The listing builds one solid part. Answer for the finished solid, in the listing's coordinates (mm). A direction names the side the tool comes from. Give positions to 0.01 mm unless a question says otherwise; leave off trailing zeros. Loops run counter-clockwise (first coordinate to the right, second up) from the corner with the lowest first, then second, coordinate; pieces in that order, holes last.
Item 1: Each of these flat-tipped pins is pushed along its axis until it touches: pin 1 Ø6 at (x, z) = (-109, 26.5) entering from -Y; pin 2 Ø10 at (x, y) = (-134.5, 146) entering from +Z; pin 3 Ø6.5 at (y, z) = (-149.5, 4.5) entering from +X. Where does it stop, or does it pass through?
Item 2: Section C-C, the plane x = 77 is taken. Give the vertices of the cut face in (y, z).
Item 3: A tool of negligible diameter and unlimited length cuts with its end or side. For faces 4 (the face through (12.7, 149, 6)), 5 (the face through (-2, -117, -25.4)), 6 (the face through (-2, 118, -25.4)), 7 (the face through (-91.315, -114.144, -12.522)), from which of +Z, -Z, +X, -X, +Y, -Y can it reach the whole face along a straight path? Write none if from no direction.
Item 4: Consider line 1 along Z through (x, y) = (-161, 0); line 2 along Y through (x, z) = (-107.5, 90.5); line 3 along Y through (x, z) = (-145, 133). Determine where each line is inside the solid, lowest interval first.
Item 5: Section A-A, the plane z = 133.35 is taken. Give the vertices of the cut face in (x, y), and give its area (3 significant figures).
Item 6: Section D-D, the plane y = 0 is taken. Give the vertices of the cut face in (x, z).
Item 7: The mould has two halves that part along X. Classify faces 1 (the face through (-58.1, -149.4, 83.5)), 2 (the face through (156.335, -114.144, -12.522)), 3 (the face through (-82, -158.75, 58)): pulls with the +X half, pulls with the -X half, needs draft (parallel to the pull), parting line crosses it, or undercut.
Item 8: Section B-B, the plane y = 114.3 is taken. Give the vertices of the cut face in (x, z).
from build123d import *

# Parameters (mm, degrees)
F0_W           = 342.9
F0_H           = 330.2
F1_DEPTH       = 25.4
F2_W           = 342.9
F2_H           = 139.7
F3_DEPTH       = 6.35
F4_W           = 25.4
F4_H           = 304.8
F5_DEPTH       = 215.9
F7_D           = 127
F7_CBORE_D     = 139.7
F7_CBORE_DEPTH = 12.7
F9_DEPTH       = 1.524
F11_D          = 10.71626
F12_W          = 152.4
F12_H          = 19.05
F13_DEPTH      = 152.4
F14_SIZE       = 139.7


with BuildPart() as f1:
    # F0 (on Top) → F1 (new body)
    with BuildSketch(Plane.XY):
        Rectangle(F0_W, F0_H)
        with BuildLine():
            Line((-98.425, -121.412), (-117.475, -121.412))
            ThreePointArc((-117.475, -121.412), (-124.587, -114.3), (-117.475, -107.188))
            Line((-117.475, -107.188), (-98.425, -107.188))
            ThreePointArc((-98.425, -107.188), (-91.313, -114.3), (-98.425, -121.412))
        make_face(mode=Mode.SUBTRACT)
        with BuildLine():
            Line((149.225, -121.412), (130.175, -121.412))
            ThreePointArc((130.175, -121.412), (123.063, -114.3), (130.175, -107.188))
            Line((130.175, -107.188), (149.225, -107.188))
            ThreePointArc((149.225, -107.188), (156.337, -114.3), (149.225, -121.412))
        make_face(mode=Mode.SUBTRACT)
        with BuildLine():
            Line((-98.425, 107.188), (-117.475, 107.188))
            ThreePointArc((-117.475, 107.188), (-124.587, 114.3), (-117.475, 121.412))
            Line((-117.475, 121.412), (-98.425, 121.412))
            ThreePointArc((-98.425, 121.412), (-91.313, 114.3), (-98.425, 107.188))
        make_face(mode=Mode.SUBTRACT)
        with BuildLine():
            Line((149.225, 107.188), (130.175, 107.188))
            ThreePointArc((130.175, 107.188), (123.063, 114.3), (130.175, 121.412))
            Line((130.175, 121.412), (149.225, 121.412))
            ThreePointArc((149.225, 121.412), (156.337, 114.3), (149.225, 107.188))
        make_face(mode=Mode.SUBTRACT)
    extrude(amount=-F1_DEPTH)

    # F2 (on face) → F3 (join)
    with BuildSketch(Plane(origin=(0, 0, -25.4), x_dir=(1, 0, 0), z_dir=(0, 0, -1))):
        Rectangle(F2_W, F2_H)
    extrude(amount=F3_DEPTH)

    # F4 (on face) → F5 (join)
    with BuildSketch(Plane.XY):
        with Locations((-152.4, 0)):
            Rectangle(F4_W, F4_H)
    extrude(amount=F5_DEPTH)

    # F7 (through all)
    with Locations(Plane(origin=(-165.1, 0, 0), x_dir=(0, -1, 0), z_dir=(-1, 0, 0))):
        with Locations((0, 133.35)):
            CounterBoreHole(F7_D / 2, F7_CBORE_D / 2, F7_CBORE_DEPTH)

    # F8 (on face) → F9 (cut)
    with BuildSketch(Plane.YZ.offset(-139.7)):
        with BuildLine():
            Line((0, 31.75), (50.8, 31.75))
            ThreePointArc((50.8, 31.75), (68.7605122421, 39.1894877579), (76.2, 57.15))
            Line((76.2, 57.15), (76.2, 215.9))
            Line((76.2, 215.9), (0, 215.9))
            Line((0, 215.9), (0, 31.75))
        make_face()
        with BuildLine():
            Line((-50.8, 31.75), (0, 31.75))
            Line((0, 31.75), (0, 215.9))
            Line((0, 215.9), (-76.2, 215.9))
            Line((-76.2, 215.9), (-76.2, 57.15))
            ThreePointArc((-76.2, 57.15), (-68.7605122421, 39.1894877579), (-50.8, 31.75))
        make_face()
    extrude(amount=-F9_DEPTH, mode=Mode.SUBTRACT)

    # F11 (through all)
    with Locations(Plane.YZ.offset(-141.224)):
        with Locations((57.2940340524, 190.6440340524), (57.2940340524, 76.0559659476), (-57.2940340524, 76.0559659476), (-57.2940340524, 190.6440340524)):
            Hole(F11_D / 2)

    # F12 (on face) → F13 (join)
    with BuildSketch(Plane.XY):
        with Locations((-63.5, 149.225)):
            Rectangle(F12_W, F12_H)
        with Locations((-63.5, -149.225)):
            Rectangle(F12_W, F12_H)
    extrude(amount=F13_DEPTH)

    # F14
    f14_edges = [f1.edges().sort_by_distance(p)[0] for p in [
        (12.7, 149.225, 152.4),
        (12.7, -149.225, 152.4),
    ]]
    chamfer(f14_edges, length=F14_SIZE)


solid = f1.part
Worked answers:
1. pin 1: stops at y = -158.75
1. pin 2: stops at z = 152.4
1. pin 3: stops at x = 12.7
2. outline: (-165.1, -25.4) - (-69.85, -25.4) - (-69.85, -31.75) - (69.85, -31.75) - (69.85, -25.4) - (165.1, -25.4) - (165.1, 0) - (-165.1, 0) - close
3. face 4: +Z, +X, +Y, -Y
3. face 5: -Z, +X, -X, -Y
3. face 6: -Z, +X, -X, +Y
3. face 7: +Z, -Z
4. line 1: z = -31.75 to 63.5, 203.2 to 215.9
4. line 2: y = -158.75 to -139.7, 139.7 to 158.75
4. line 3: y = -152.4 to -63.5, 63.5 to 152.4
5. outline: (-165.1, -152.4) - (-139.7, -152.4) - (-139.7, -158.75) - (-107.95, -158.75) - (-107.95, -139.7) - (-139.7, -139.7) - (-139.7, -76.2) - (-141.22, -76.2) - (-141.22, -63.5) - (-152.4, -63.5) - (-152.4, -69.85) - (-165.1, -69.85) - close; (-165.1, 69.85) - (-152.4, 69.85) - (-152.4, 63.5) - (-141.22, 63.5) - (-141.22, 76.2) - (-139.7, 76.2) - (-139.7, 139.7) - (-107.95, 139.7) - (-107.95, 158.75) - (-139.7, 158.75) - (-139.7, 152.4) - (-165.1, 152.4) - close
5. area: 5,530 mm2
6. outline: (-171.45, -31.75) - (171.45, -31.75) - (171.45, 0) - (-139.7, 0) - (-139.7, 31.75) - (-141.22, 31.75) - (-141.22, 69.85) - (-152.4, 69.85) - (-152.4, 63.5) - (-165.1, 63.5) - (-165.1, 0) - (-171.45, 0) - close; (-165.1, 203.2) - (-152.4, 203.2) - (-152.4, 196.85) - (-141.22, 196.85) - (-141.22, 215.9) - (-165.1, 215.9) - close
7. face 1: pulls with the +X half
7. face 2: undercut
7. face 3: needs draft
8. outline: (-171.45, -25.4) - (-124.59, -25.4) - (-124.59, 0) - (-139.7, 0) - (-139.7, 215.9) - (-165.1, 215.9) - (-165.1, 0) - (-171.45, 0) - close; (-91.31, -25.4) - (123.06, -25.4) - (123.06, 0) - (-91.31, 0) - close; (156.34, -25.4) - (171.45, -25.4) - (171.45, 0) - (156.34, 0) - close
